Source: CAD feature listing. Evaluate the final solid. Frame: model axes, mm. Face numbers are marked on the shaded views. A direction names the side the tool comes from. Round coordinates to 2 decimals unless told otherwise and drop trailing zeros. Order: outer loops, then holes, each group sorted by start corner. A loop starts at its lowest first (then second) coordinate and runs counter-clockwise, first axis right, second up. Notation, with made-up numbers: M 53,-10 L 84,-10 A37 ccw 84,29 Z; hole C 19,31.5 d2. An arc over 180 degrees is marked long. Use one line per item in the form item = value. Start each with the question number.
Q1. Section A-A (z = 3). Return the cut outline in (x, y), plus the area to 3 significant figures.
Q2. Contact query for flat-ended pins moving along their axis: pin 1 (1 mm diameter, centred on y = -4, z = 2.5, fed in from -X); pin 2 (3 mm diameter, centred on y = 3.5, z = 0.5, fed in from -X); pin 3 (3 mm diameter, centred on x = 20.5, z = 3.5, fed in from +Y). Output: stop coordinate, or through.
Q3. Material intervals for probe 1 along X at (y, z) = (-2.25, 1.25); probe 2 along X at (y, z) = (-3.75, 1); probe 3 along Y at (x, z) = (56.5, 3), sorted ascending.
Q4. Section D-D (x = 50.5). Return the cut outline in (y, z).
Q5. Section C-C (y = 0). Return the cut outline in (x, z), plus the area to 3 significant figures.
Q6. Section B-B (x = 8). Return the cut outline in (y, z), plus the area to 3 significant figures.
Q7. Pull-direction query (X, two-part tool) for the marked faces 4, 5 and 6; classes: pulls with the +X half, pulls with the -X half, needs draft (parallel to the pull), parting line crosses it, or undercut.
Q8. Reachability of the marked faces 1, 2 and 3 from +Z, -Z, +X, -X, +Y, -Y: full face, straight path, thin tool, end or side. Return the list, or none.
from build123d import *

# Parameters (mm, degrees)
BOSS_EXTRUDE2_DEPTH = 6
FILLET2_R           = 25
CHAMFER2_SIZE       = 1


with BuildPart() as part:
    # Sketch7 → Boss-Extrude2 (new body)
    with BuildSketch(Plane(origin=(0, 0, 0), x_dir=(-1, 0, 0), z_dir=(0, 0, -1))):
        with BuildLine():
            Line((-78.562859207, -4), (-13.437140793, -4))
            ThreePointArc((-13.437140793, -4), (-1.25, 0), (-13.437140793, 4))
            Line((-13.437140793, 4), (-78.562859207, 4))
            ThreePointArc((-78.562859207, 4), (-90.75, 0), (-78.562859207, -4))
        make_face()
    extrude(amount=-BOSS_EXTRUDE2_DEPTH)

    # Sketch10 → Cut-Revolve3 (revolve, cut)
    with BuildSketch(Plane(origin=(0, 0, 0), x_dir=(1, 0, 0), z_dir=(0, 1, 0))):
        with BuildLine():
            Line((88.787744772, 0), (84, 0))
            Line((84, 0), (84, -6))
            Line((84, -6), (89.618941181, -6))
            ThreePointArc((89.618941181, -6), (89.199640564, -5.772372891), (89.162116695, -5.296747967))
            ThreePointArc((89.162116695, -5.296747967), (89.635940078, -2.601654121), (88.787744772, 0))
        make_face()
    revolve(axis=Axis((84, 0, 0), (0, 0, 1)), mode=Mode.SUBTRACT)

    # Sketch13 → Cut-Revolve4 (revolve, cut)
    with BuildSketch(Plane(origin=(0, 0, 0), x_dir=(1, 0, 0), z_dir=(0, 1, 0))):
        with BuildLine():
            Line((12.787744772, 0), (8, 0))
            Line((8, 0), (8, -6))
            Line((8, -6), (13.618941181, -6))
            ThreePointArc((13.618941181, -6), (13.199640564, -5.772372891), (13.162116695, -5.296747967))
            ThreePointArc((13.162116695, -5.296747967), (13.635940078, -2.601654121), (12.787744772, 0))
        make_face()
    revolve(axis=Axis((8, 0, 0), (0, 0, 1)), mode=Mode.SUBTRACT)

    # Fillet2
    fillet2_edges = [part.edges().sort_by_distance(p)[0] for p in [
        (13.437140793, -4, 3),
        (78.562859207, -4, 3),
        (78.562859207, 4, 3),
        (13.437140793, 4, 3),
    ]]
    fillet(fillet2_edges, radius=FILLET2_R)

    # Chamfer2
    chamfer2_edges = [part.edges().sort_by_distance(p)[0] for p in [
        (46, 4, 6),
        (90.75, 0, 6),
        (46, -4, 6),
        (1.25, 0, 6),
        (76.277322741, 4.547329985, 6),
        (15.722677259, -4.547329985, 6),
        (76.277322741, -4.547329985, 6),
        (15.722677259, 4.547329985, 6),
    ]]
    chamfer(chamfer2_edges, length=CHAMFER2_SIZE)


solid = part.part
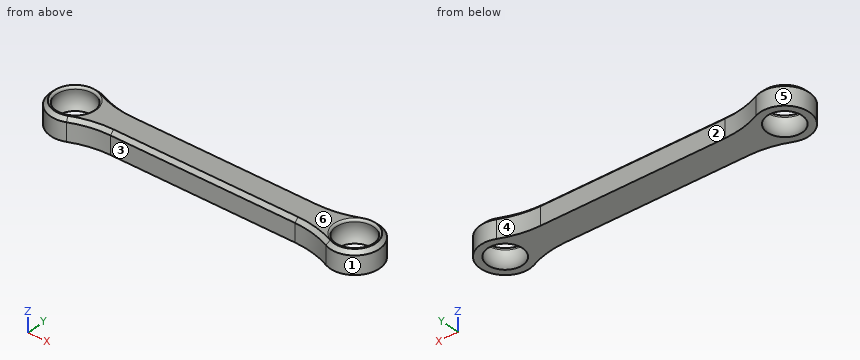
Results list:
q1.outline = M 10.75,-6.17 A25 cw 20.93,-4 L 71.07,-4 A25 cw 81.25,-6.17 A6.75 ccw long 81.25,6.17 A25 cw 71.07,4 L 20.93,4 A25 cw 10.75,6.17 A6.75 ccw long Z; hole C 8,0 d11.3; hole C 84,0 d11.3
q1.area = 608 mm2
q2.pin_1 = 2.23
q2.pin_2 = 1.55
q2.pin_3 = 4.07
q3.probe_1 = 1.64 to 3.12, 12.88 to 79.12, 88.88 to 90.36
q3.probe_2 = 2.39 to 4.28, 11.72 to 80.28, 87.72 to 89.61
q3.probe_3 = -4 to 4
q4.outline = M -4,0 L 4,0 L 4,5 L 3,6 L -3,6 L -4,5 Z
q5.outline = M 1.25,0 L 3.21,0 A5.65 cw 2.84,5.3 A0.5 ccw 2.38,6 L 2.25,6 L 1.25,5 Z; M 12.79,0 L 79.21,0 A5.65 cw 78.84,5.3 A0.5 ccw 78.38,6 L 13.62,6 A0.5 ccw 13.16,5.3 A5.65 cw Z; M 88.79,0 L 90.75,0 L 90.75,5 L 89.75,6 L 89.62,6 A0.5 ccw 89.16,5.3 A5.65 cw Z
q5.area = 406 mm2
q6.outline = M -6.75,0 L -4.79,0 A5.65 cw -5.16,5.3 A0.5 ccw -5.62,6 L -5.75,6 L -6.75,5 Z; M 4.79,0 L 6.75,0 L 6.75,5 L 5.75,6 L 5.62,6 A0.5 ccw 5.16,5.3 A5.65 cw Z
q6.area = 15.2 mm2
q7.face_4 = undercut
q7.face_5 = undercut
q7.face_6 = needs draft
q8.face_1 = +Z, -Z
q8.face_2 = +Z, -Z, +Y
q8.face_3 = +Z, -Z, -Y
